```python
from build123d import *

# Parameters (mm, degrees)
F1_DEPTH = 10
F2_W     = 2
F2_H     = 6
F3_DEPTH = 9.001


with BuildPart() as f1:
    # F0 (on Front) → F1 (new body)
    with BuildSketch(Plane.XZ):
        Polygon((-6, 9), (-10, 9), (-10, 0), (0, 0), align=None)
    extrude(amount=-F1_DEPTH)

    # F2 (on face) → F3 (cut, through all)
    with BuildSketch(Plane.XY.offset(9)):
        with Locations((-9, 5)):
            Rectangle(F2_W, F2_H)
    extrude(amount=-F3_DEPTH, mode=Mode.SUBTRACT)

    # F4 (on Right) → F5 (join, up to the next surface of F1)
    with BuildSketch(Plane.YZ):
        Polygon((0, 0), (10, 0), (5, 5), align=None)
    extrude(until=Until.NEXT, dir=(-1, 0, 0))


solid = f1.part
```
Input: part model. Units: mm. Frame: model coordinates. A direction names the side the tool comes from. Give positions to 0.01 mm unless a question says otherwise; leave off trailing zeros. Order: outer loops, then holes, each group sorted by start corner. A loop starts at its lowest first (then second) coordinate and runs counter-clockwise, first axis right, second up.
1. Section B-B on x = -1.5. Return the cut outline in (y, z).
Derived:
outline: (0, 0) - (10, 0) - (10, 2.25) - (7.75, 2.25) - (5, 5) - (2.25, 2.25) - (0, 2.25) - close
2. Reachability of faces 4 (the flat face through (0, 5, 2)), 5 (the flat face through (-8, 5, 5)), 6 (the flat face through (-3.6, 4.9, 5.4)), 7 (the flat face through (-1, 3, 3)) from +Z, -Z, +X, -X, +Y, -Y: full face, straight path, thin tool, end or side. Return the list, or none.
Derived:
face 4: +Z, -Z, +X, +Y, -Y
face 5: +Z, -Z, -X
face 6: +Z, +X
face 7: +Z, +X, -Y
3. Pin query (flat end, axial travel): pin 1 (2 mm diameter, centred on y = 2, z = 6, fed in from +X); pin 2 (1.8 mm diameter, centred on y = 3.5, z = 4.5, fed in from -X); pin 3 (4 mm diameter, centred on x = -1.5, y = 2, fed in from +Z). Return the tip coordinate at first contact, or that it passes through.
Derived:
pin 1: stops at x = -3.33
pin 2: stops at x = -8
pin 3: stops at z = 5.25
4. Mould query, pull axis Y, two halves, no side actions, for faces 1 (the flat face through (-9, 2, 5)), 2 (the flat face through (-1, 6, 4)), 3 (the flat face through (-10, 1, 5)). Classes: released by +Y, released by -Y, zero draft, split by the parting line, or undercut.
Derived:
face 1: undercut
face 2: released by +Y
face 3: zero draft
5. Material intervals for L1, parallel to Y at x = -8.5, z = 5; L2, parallel to X at y = 0.5, z = 5; L3, parallel to X at y = 2.5, z = 8.5, sorted ascending.
Derived:
L1: y = 0 to 2, 8 to 10
L2: x = -10 to -3.33
L3: x = -8 to -5.67
6. Section A-A on x = -8.75. Return the cut outline in (y, z), and give its area (3 significant figures).
Derived:
outline: (0, 0) - (2, 0) - (2, 9) - (0, 9) - close; (8, 0) - (10, 0) - (10, 9) - (8, 9) - close
area: 36.0 mm2
7. Section D-D on z = 4.5. Return the cut outline in (x, y), and give its area (3 significant figures).
Derived:
outline: (-10, 0) - (-3, 0) - (-3, 4.5) - (0, 4.5) - (0, 5.5) - (-3, 5.5) - (-3, 10) - (-10, 10) - (-10, 8) - (-8, 8) - (-8, 2) - (-10, 2) - close
area: 61.0 mm2
8. Section C-C on y = 7.75. Return the cut outline in (x, z), and give its area (3 significant figures).
Derived:
outline: (-8, 0) - (0, 0) - (0, 2.25) - (-1.5, 2.25) - (-6, 9) - (-8, 9) - close
area: 46.7 mm2
